Design review of the part shown in the three views and the two pictorial views. Dimensions are in mm from the part's minimum x, y and z. A direction names the side the tool comes from. Coordinates: 2 decimals unless noted, no trailing zeros. Order: outer loops, then holes, each group sorted by start corner. A loop starts at its lowest first (then second) coordinate and runs counter-clockwise, first axis right, second up. Notation, with made-up numbers: (32.5, -30) -> (73.5, -30) arc R18 ccw to (73.5, -18) -> close; hole circle Ø2 at (-20.75, -37). An arc over 180 degrees is marked (long way). Write item = value, one per line. Start each with the question number.
1) Machinability: for the marked faces 1 and 2, which of the approach directions +Z, -Z, +X, -X, +Y, -Y give a long, thin tool a straight path to every point of the face, cutting with its end or side? Answer none if there is none.
2) Consider section D-D on x = 2.5. Give the boundary of the cut face in (y, z), and give its area (3 significant figures).
3) Consider section B-B on y = 8. Give the boundary of the cut face in (x, z).
4) Insertion check: pin 1 Ø3.5 at (y, z) = (3.5, 5.5) entering from -X. The pin has a flat end and moves straight along its axis. Give the tip position at first contact, or say it passes through.
5) Wall thickness on probe 1 along X at (y, z) = (8.85, 5); probe 2 along Z at (x, y) = (2.5, 9); probe 3 along Y at (x, z) = (15, 1.25): over which ranges is each line inside the solid? List them lowest first. Write a range as [from, to].
6) Draft analysis for pull direction Y (two halves, no side actions). For the marked faces 3, 4 and 5, state which applies: +Y half, -Y half, draft (parallel to the pull), parting line (faces both ways), or undercut.
7) Consider section C-C on z = 6. Give the boundary of the cut face in (x, y), and give its area (3 significant figures).
8) Consider section A-A on x = 32.5. Give the boundary of the cut face in (y, z), and give its area (3 significant figures).
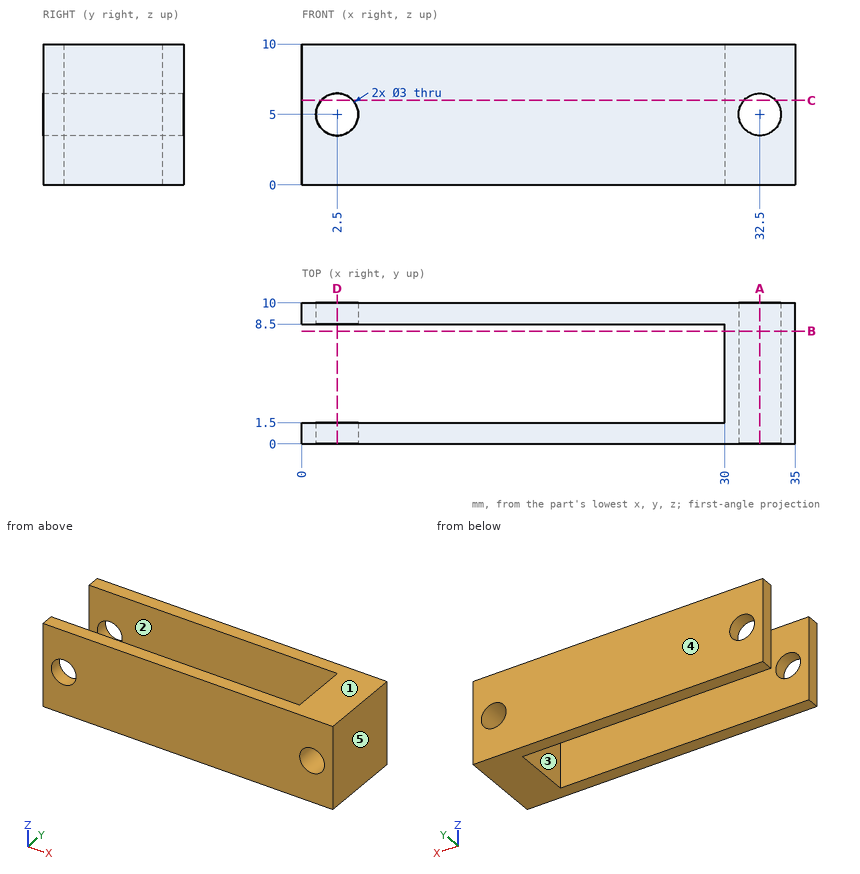
Answer sheet:
q1.face_1 = +Z, +X, -X, +Y, -Y
q1.face_2 = +Z, -Z, -X
q2.outline = (0, 0) -> (1.5, 0) -> (1.5, 3.5) -> (0, 3.5) -> close; (0, 6.5) -> (1.5, 6.5) -> (1.5, 10) -> (0, 10) -> close; (8.5, 0) -> (10, 0) -> (10, 3.5) -> (8.5, 3.5) -> close; (8.5, 6.5) -> (10, 6.5) -> (10, 10) -> (8.5, 10) -> close
q2.area = 21.0 mm2
q3.outline = (30, 0) -> (35, 0) -> (35, 10) -> (30, 10) -> close; hole circle Ø3 at (32.5, 5)
q4.pin_1 = 30
q5.probe_1 = [0, 1], [4, 31], [34, 35]
q5.probe_2 = [0, 3.5], [6.5, 10]
q5.probe_3 = [0, 1.5], [8.5, 10]
q6.face_3 = undercut
q6.face_4 = +Y half
q6.face_5 = draft
q7.outline = (0, 0) -> (1.38, 0) -> (1.38, 1.5) -> (0, 1.5) -> close; (0, 8.5) -> (1.38, 8.5) -> (1.38, 10) -> (0, 10) -> close; (3.62, 0) -> (31.38, 0) -> (31.38, 10) -> (3.62, 10) -> (3.62, 8.5) -> (30, 8.5) -> (30, 1.5) -> (3.62, 1.5) -> close; (33.62, 0) -> (35, 0) -> (35, 10) -> (33.62, 10) -> close
q7.area = 111 mm2
q8.outline = (0, 0) -> (10, 0) -> (10, 3.5) -> (0, 3.5) -> close; (0, 6.5) -> (10, 6.5) -> (10, 10) -> (0, 10) -> close
q8.area = 70.0 mm2
